The listing builds one solid part. Answer for the finished solid, in the listing's coordinates (mm). A direction names the side the tool comes from. Coordinates: 2 decimals unless noted, no trailing zeros. Loops run counter-clockwise (first coordinate to the right, second up) from the corner with the lowest first, then second, coordinate; pieces in that order, holes last. Notation, with made-up numbers: (-4, 4) - (53, 4) arc R21 ccw to (53, 8) - close; hole circle Ø11 at (12.5, -9.5). An arc over 180 degrees is marked (long way). Return JSON: item names as keys, results as strings. Group by question number.
1. Section A-A (x = -12) is taken. Write down the section's boundary in (y, z), and give its area (3 significant figures).
2. Section C-C (z = 9) is taken. Write down the section's boundary in (x, y), and give its area (3 significant figures).
3. Which of the six approach directions +Z, -Z, +X, -X, +Y, -Y give full straight-line access (tool end or side, diameter ignored) to faces 1 (the face through (0, -123, -22.5)), 2 (the face through (-25, -123, 0))?
4. Section B-B (y = -103) is taken. Write down the section's boundary in (x, z).
5. The mould has two halves that part along X. Classify faces 3 (the face through (-2, 0, -24)), 4 (the face through (-22.5, -123, 0)), 5 (the face through (23.859, -123.25, 23.797)), 6 (the face through (-23.797, -123.25, 23.859)): pulls with the +X half, pulls with the -X half, needs draft (parallel to the pull), parting line crosses it, or undercut.
6. Find the intervals of material crossed by line 1 along X through (y, z) = (-142, -10); line 2 along X through (y, z) = (-36.5, 22), in increasing order.
```python
from build123d import *

# Parameters (mm, degrees)
F1_DEPTH = 250


# Not quite as in the source:
# - a feature names something its author has since deleted; it is built from what else it names


with BuildPart() as f1:
    # F0 (on Front) → F1 (new body)
    with BuildSketch(Plane.XZ):
        with BuildLine():
            Line((21, 25), (-21, 25))
            ThreePointArc((-21, 25), (-23.8284271247, 23.8284271247), (-25, 21))
            Line((-25, 21), (-25, -21))
            ThreePointArc((-25, -21), (-23.8284271247, -23.8284271247), (-21, -25))
            Line((-21, -25), (21, -25))
            ThreePointArc((21, -25), (23.8284271247, -23.8284271247), (25, -21))
            Line((25, -21), (25, 21))
            ThreePointArc((25, 21), (23.8284271247, 23.8284271247), (21, 25))
        make_face()
        with BuildLine():
            ThreePointArc((-22.5, 21), (-22.0606601718, 22.0606601718), (-21, 22.5))
            Line((-21, 22.5), (21, 22.5))
            ThreePointArc((21, 22.5), (22.0606601718, 22.0606601718), (22.5, 21))
            Line((22.5, 21), (22.5, -21))
            ThreePointArc((22.5, -21), (22.0606601718, -22.0606601718), (21, -22.5))
            Line((21, -22.5), (-21, -22.5))
            ThreePointArc((-21, -22.5), (-22.0606601718, -22.0606601718), (-22.5, -21))
            Line((-22.5, -21), (-22.5, 21))
        make_face(mode=Mode.SUBTRACT)
    extrude(amount=F1_DEPTH)


solid = f1.part
```
The answers:
{
 "1": {"outline": "(-250, -25) - (0, -25) - (0, -22.5) - (-250, -22.5) - close; (-250, 22.5) - (0, 22.5) - (0, 25) - (-250, 25) - close", "area": "1,250 mm2"},
 "2": {"outline": "(-25, -250) - (-22.5, -250) - (-22.5, 0) - (-25, 0) - close; (22.5, -250) - (25, -250) - (25, 0) - (22.5, 0) - close", "area": "1,250 mm2"},
 "3": {"face 1": "+Y, -Y", "face 2": "+Z, -Z, -X, +Y, -Y"},
 "4": {"outline": "(-25, -21) arc R4 ccw to (-21, -25) - (21, -25) arc R4 ccw to (25, -21) - (25, 21) arc R4 ccw to (21, 25) - (-21, 25) arc R4 ccw to (-25, 21) - close; hole (-22.5, -21) arc R1.5 ccw to (-21, -22.5) - (21, -22.5) arc R1.5 ccw to (22.5, -21) - (22.5, 21) arc R1.5 ccw to (21, 22.5) - (-21, 22.5) arc R1.5 ccw to (-22.5, 21) - close"},
 "5": {"face 3": "needs draft", "face 4": "undercut", "face 5": "pulls with the +X half", "face 6": "pulls with the -X half"},
 "6": {"line 1": "x = -25 to -22.5, 22.5 to 25", "line 2": "x = -24.87 to -22.12, 22.12 to 24.87"}
}
